Here's how the part is built. I have some questions about the finished solid (model axes, mm). Round coordinates to 2 decimals unless told otherwise and drop trailing zeros. Write each loop counter-clockwise with the first axis right and the second up, starting at its lowest first coordinate (ties: lowest second). Pieces come first, ordered by that corner, then holes. Notation, with made-up numbers: (8, -19) - (24, -19) arc R16 ccw to (24, 4) - close; hole circle Ø8 at (10, 9). An arc over 180 degrees is marked (long way). Use one line per item in the form item = value. Start each with the question number.
1. I want a section at A-A, the plane z = 14.5. List the corners of the cut face in (x, y) for me.
2. I want a section at C-C, the plane x = -72.5. List the corners of the cut face in (y, z) for me.
3. I want a section at B-B, the plane y = -34. List the corners of the cut face in (x, z) for me.
4. If I drill on line 1 along X through (y, z) = (53.5, 17.5); line 2 along X through (y, z) = (61, 14.75); line 3 along Y through (x, z) = (20.5, 20), over which ranges is the centre line in solid material (lowest first)?
5. Will these pins go through, and if not, where does the flat tip stop? pin 1 (4 mm diameter, centred on x = 6.5, z = 3, fed in from -Y); pin 2 (1 mm diameter, centred on y = 28, z = 21.5, fed in from +X); pin 3 (2 mm diameter, centred on y = 46, z = 20.5, fed in from +X).
```python
from build123d import *

# Parameters (mm, degrees)
F0_R     = 56.338537
F0_W     = 43.072939
F0_H     = 0.103983
F0_W_2   = 40.760524
F0_H_2   = 0.144385
F1_DEPTH = 25.4


with BuildPart() as f1:
    # F0 (on Top) → F1 (new body)
    with BuildSketch(Plane.XY):
        with Locations((-24.527786, 10.620722)):
            Circle(F0_R)
        with Locations((-35.37745, 6.090215)):
            Rectangle(F0_W, F0_H, mode=Mode.SUBTRACT)
        with Locations((-34.221243, 33.007942)):
            Rectangle(F0_W_2, F0_H_2, mode=Mode.SUBTRACT)
    extrude(amount=F1_DEPTH)


solid = f1.part
```
Model answer:
q1.outline = circle Ø112.68 at (-24.53, 10.62); hole (-56.91, 6.04) - (-13.84, 6.04) - (-13.84, 6.14) - (-56.91, 6.14) - close; hole (-54.6, 32.94) - (-13.84, 32.94) - (-13.84, 33.08) - (-54.6, 33.08) - close
q2.outline = (-18.92, 0) - (40.16, 0) - (40.16, 25.4) - (-18.92, 25.4) - close
q3.outline = (-58.92, 0) - (9.87, 0) - (9.87, 25.4) - (-58.92, 25.4) - close
q4.line_1 = -61.07 to 12.02
q4.line_2 = -49.75 to 0.69
q4.line_3 = -23.24 to 44.48
q5.pin_1 = -37.66
q5.pin_2 = 29.22
q5.pin_3 = 20.11
